Geometry check sheet. Reference: the model listing, model coordinates, mm. Face numbers are marked on the shaded views. A direction names the side the tool comes from. Give positions to 0.01 mm unless a question says otherwise; leave off trailing zeros. Write each loop counter-clockwise with the first axis right and the second up, starting at its lowest first coordinate (ties: lowest second). Pieces come first, ordered by that corner, then holes. Notation, with made-up numbers: (0.5, 35.5) -> (11.5, 35.5) arc R27 ccw to (11.5, 59.5) -> close; hole circle Ø9 at (13.5, 5). An arc over 180 degrees is marked (long way). Write item = value, one per line. Start each with the question number.
1. Depth check by flat-ended pin: P1, Ø5.5, axis at x = -21, y = -2, coming from the -Z side; P2, Ø6, axis at y = 4, z = 3.5, coming from the -X side; P3, Ø4, axis at x = 21.25, y = -3.75, coming from the +Z side. Enter the tip coordinate at first touch or a pass-through.
2. Cross-section at C-C, the plane x = -8.5. Record the cut outline in (y, z), plus the area to 3 significant figures.
3. Set-up check for the marked faces 1, 2, 3 and 4: record each of +Z, -Z, +X, -X, +Y, -Y from which the full face is reachable in a straight line by a thin tool's end or side.
4. Cross-section at B-B, the plane y = 0. Record the cut outline in (x, z), plus the area to 3 significant figures.
5. Cross-section at D-D, the plane z = 15. Record the cut outline in (x, y), plus the area to 3 significant figures.
6. Cross-section at A-A, the plane x = 21.25. Record the cut outline in (y, z).
7. Thickness scan on line 1 along Y through (x, z) = (21.25, 21.45); line 2 along X through (y, z) = (6.5, 25.5); line 3 along Z through (x, y) = (17, -5). Record the ranges inside material, lowest first.
```python
from build123d import *

# Parameters (mm, degrees)
SZKIC1_W                    = 35
SZKIC1_H                    = 15
DODANIE_WYCI_GNI_CIE1_DEPTH = 20.5
DODANIE_WYCI_GNI_CIE2_DEPTH = 2
SZKIC3_W                    = 35
SZKIC3_H                    = 15
DODANIE_WYCI_GNI_CIE3_DEPTH = 6.7
SZKIC4_R                    = 3
DODANIE_WYCI_GNI_CIE4_DEPTH = 4.8


with BuildPart() as part:
    # Szkic1 → Dodanie-wyciągnięcie1 (new body)
    with BuildSketch(Plane.XY):
        Rectangle(SZKIC1_W, SZKIC1_H)
    extrude(amount=DODANIE_WYCI_GNI_CIE1_DEPTH)

    # Szkic2 → Dodanie-wyciągnięcie2 (add)
    with BuildSketch(Plane.XY.offset(20.5)):
        with BuildLine():
            Line((-24.2, 7.5), (24.2, 7.5))
            Line((24.2, 7.5), (24.2, 4.5))
            Line((24.2, 4.5), (22.83113883, 4.5))
            ThreePointArc((22.83113883, 4.5), (19.5, 3.75), (22.83113883, 3))
            Line((22.83113883, 3), (24.2, 3))
            Line((24.2, 3), (24.2, -3))
            Line((24.2, -3), (22.83113883, -3))
            ThreePointArc((22.83113883, -3), (19.5, -3.75), (22.83113883, -4.5))
            Line((22.83113883, -4.5), (24.2, -4.5))
            Line((24.2, -4.5), (24.2, -7.5))
            Line((24.2, -7.5), (-24.2, -7.5))
            Line((-24.2, -7.5), (-24.2, -4.5))
            Line((-24.2, -4.5), (-22.83113883, -4.5))
            ThreePointArc((-22.83113883, -4.5), (-19.5, -3.75), (-22.83113883, -3))
            Line((-22.83113883, -3), (-24.2, -3))
            Line((-24.2, -3), (-24.2, 3))
            Line((-24.2, 3), (-22.83113883, 3))
            ThreePointArc((-22.83113883, 3), (-19.5, 3.75), (-22.83113883, 4.5))
            Line((-22.83113883, 4.5), (-24.2, 4.5))
            Line((-24.2, 4.5), (-24.2, 7.5))
        make_face()
    extrude(amount=DODANIE_WYCI_GNI_CIE2_DEPTH)

    # Szkic3 → Dodanie-wyciągnięcie3 (add)
    with BuildSketch(Plane.XY.offset(22.5)):
        Rectangle(SZKIC3_W, SZKIC3_H)
    extrude(amount=DODANIE_WYCI_GNI_CIE3_DEPTH)

    # Szkic4 → Dodanie-wyciągnięcie4 (add)
    with BuildSketch(Plane.XY.offset(29.2)):
        with Locations((-8.5, 0)):
            Circle(SZKIC4_R)
    extrude(amount=DODANIE_WYCI_GNI_CIE4_DEPTH)


solid = part.part
```
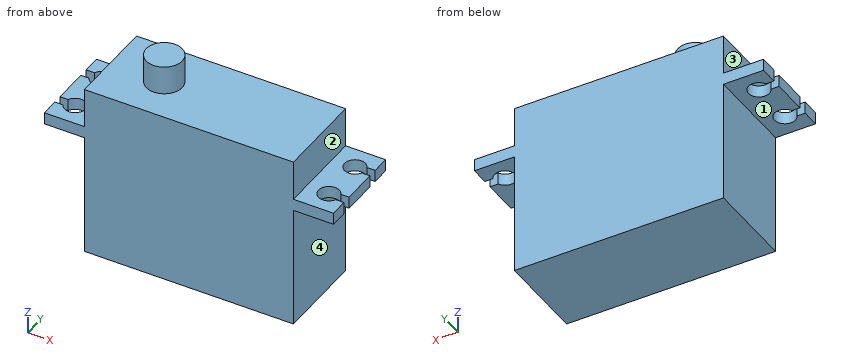
Answers:
q1.P1 = 20.5
q1.P2 = -17.5
q1.P3 = 22.5
q2.outline = (-7.5, 0) -> (7.5, 0) -> (7.5, 29.2) -> (3, 29.2) -> (3, 34) -> (-3, 34) -> (-3, 29.2) -> (-7.5, 29.2) -> close
q2.area = 467 mm^2
q3.face_1 = -Z, -X, +Y, -Y
q3.face_2 = +Z, +X, +Y, -Y
q3.face_3 = +Z, -X, +Y, -Y
q3.face_4 = -Z, +X, +Y, -Y
q4.outline = (-24.2, 20.5) -> (-17.5, 20.5) -> (-17.5, 0) -> (17.5, 0) -> (17.5, 20.5) -> (24.2, 20.5) -> (24.2, 22.5) -> (17.5, 22.5) -> (17.5, 29.2) -> (-5.5, 29.2) -> (-5.5, 34) -> (-11.5, 34) -> (-11.5, 29.2) -> (-17.5, 29.2) -> (-17.5, 22.5) -> (-24.2, 22.5) -> close
q4.area = 1,080 mm^2
q5.outline = (-17.5, -7.5) -> (17.5, -7.5) -> (17.5, 7.5) -> (-17.5, 7.5) -> close
q5.area = 525 mm^2
q6.outline = (-7.5, 20.5) -> (-5.5, 20.5) -> (-5.5, 22.5) -> (-7.5, 22.5) -> close; (-2, 20.5) -> (2, 20.5) -> (2, 22.5) -> (-2, 22.5) -> close; (5.5, 20.5) -> (7.5, 20.5) -> (7.5, 22.5) -> (5.5, 22.5) -> close
q7.line_1 = -7.5 to -5.5, -2 to 2, 5.5 to 7.5
q7.line_2 = -17.5 to 17.5
q7.line_3 = 0 to 29.2
